Here's how the part is built. I have some questions about the finished solid (model axes, mm). Face numbers are marked on the shaded views. A direction names the side the tool comes from. Round coordinates to 2 decimals unless told otherwise and drop trailing zeros. Write each loop counter-clockwise with the first axis right and the second up, starting at its lowest first coordinate (ties: lowest second). Pieces come first, ordered by that corner, then holes. Notation, with made-up numbers: (41.5, -30.5) -> (99.5, -30.5) arc R28 ccw to (99.5, 7.5) -> close; hole circle Ø5 at (45.25, 87). An arc over 180 degrees is marked (long way). Answer as CSV lines item,"result".
from build123d import *

# Parameters (mm, degrees)
BOSS_EXTRUDE2_DEPTH = 8
SKETCH3_R           = 1.25
CUT_EXTRUDE1_DEPTH  = 8
CUT_EXTRUDE2_DEPTH  = 8


with BuildPart() as part:
    # Sketch1 → Boss-Extrude2 (new body)
    with BuildSketch(Plane.XY):
        with BuildLine():
            Line((-29.531751908, 7.051775609), (-24.531751908, 7.051775609))
            Line((-24.531751908, 7.051775609), (-24.531751908, -3.948224391))
            Line((-24.531751908, -3.948224391), (-134.531751908, -3.948224391))
            Line((-134.531751908, -3.948224391), (-134.531751908, 4.051775609))
            Line((-134.531751908, 4.051775609), (-36.531751908, 4.051775609))
            ThreePointArc((-36.531751908, 4.051775609), (-35.117538345, 4.637562047), (-34.531751908, 6.051775609))
            Line((-34.531751908, 6.051775609), (-34.531751908, 14.051775609))
            Line((-34.531751908, 14.051775609), (-29.531751908, 14.051775609))
            Line((-29.531751908, 14.051775609), (-29.531751908, 11.051775609))
            ThreePointArc((-29.531751908, 11.051775609), (-31.531751908, 9.051775609), (-29.531751908, 7.051775609))
        make_face()
    extrude(amount=BOSS_EXTRUDE2_DEPTH)

    # Sketch3 → Cut-Extrude1 (cut)
    with BuildSketch(Plane(origin=(0, 4.051775609, 0), x_dir=(1, 0, 0), z_dir=(0, 1, 0))):
        with Locations(Location((-130.531751908, -4, 0), (0, 0, 270))):
            Circle(SKETCH3_R)
    extrude(amount=-CUT_EXTRUDE1_DEPTH, mode=Mode.SUBTRACT)

    # Sketch4 → Cut-Extrude2 (cut)
    with BuildSketch(Plane(origin=(0, 4.051775609, 0), x_dir=(1, 0, 0), z_dir=(0, 1, 0))):
        with BuildLine():
            Line((-115.531751908, -2.5), (-95.531751908, -2.5))
            ThreePointArc((-95.531751908, -2.5), (-94.031751908, -4), (-95.531751908, -5.5))
            Line((-95.531751908, -5.5), (-115.531751908, -5.5))
            ThreePointArc((-115.531751908, -5.5), (-117.031751908, -4), (-115.531751908, -2.5))
        make_face()
    extrude(amount=-CUT_EXTRUDE2_DEPTH, mode=Mode.SUBTRACT)


solid = part.part
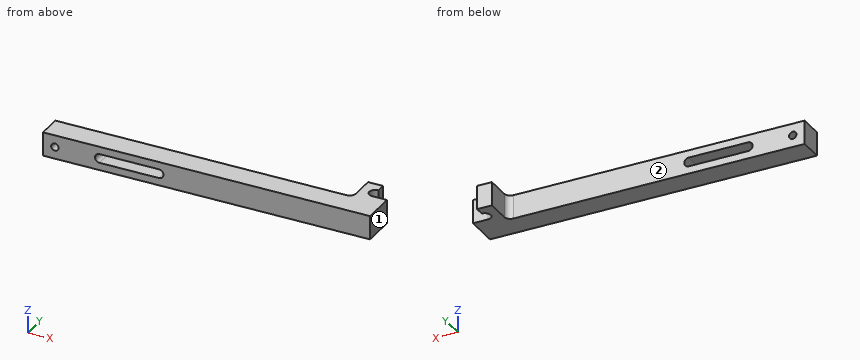
Item 1: Will these pins go through, and if not, where does the flat tip stop? pin 1 (2.5 mm diameter, centred on y = 13, z = 5.5, fed in from +X); pin 2 (4 mm diameter, centred on x = -26.5, z = 4, fed in from +Y); pin 3 (1 mm diameter, centred on y = 6, z = 3.5, fed in from -X).
Results found:
pin 1,"stops at x = -29.53"
pin 2,"stops at y = 7.05"
pin 3,"stops at x = -34.61"
Item 2: Suppose I cut it at C-C, the plane x = -71.5. List the corners of the cut face in (y, z) for me.
Results found:
outline,"(-3.95, 0) -> (4.05, 0) -> (4.05, 8) -> (-3.95, 8) -> close"
Item 3: Suppose I cut it at D-D, the plane y = 8.5. List the corners of the cut face in (x, z) for me.
Results found:
outline,"(-34.53, 0) -> (-31.45, 0) -> (-31.45, 8) -> (-34.53, 8) -> close"
Item 4: For the marked faces 1 and 2, which set-ups out of +Z, -Z, +X, -X, +Y, -Y let a thin tool reach every point of the face, with its end or its side?
Results found:
face 1,"+Z, -Z, +X, +Y, -Y"
face 2,"+Z, -Z, -X, +Y"
Item 5: Suppose I cut it at B-B, the plane y = 1. List the corners of the cut face in (x, z) for me, then the cut area to 3 significant figures.
Results found:
outline,"(-134.53, 0) -> (-24.53, 0) -> (-24.53, 8) -> (-134.53, 8) -> close; hole circle Ø2.5 at (-130.53, 4); hole (-115.53, 2.5) -> (-95.53, 2.5) arc R1.5 ccw to (-95.53, 5.5) -> (-115.53, 5.5) arc R1.5 ccw to start"
area,"808 mm²"
Item 6: Suppose I cut it at A-A, the plane z = 4. List the corners of the cut face in (x, y) for me.
Results found:
outline,"(-134.53, -3.95) -> (-131.78, -3.95) -> (-131.78, 4.05) -> (-134.53, 4.05) -> close; (-129.28, -3.95) -> (-117.03, -3.95) -> (-117.03, 4.05) -> (-129.28, 4.05) -> close; (-94.03, -3.95) -> (-24.53, -3.95) -> (-24.53, 7.05) -> (-29.53, 7.05) arc R2 cw to (-29.53, 11.05) -> (-29.53, 14.05) -> (-34.53, 14.05) -> (-34.53, 6.05) arc R2 cw to (-36.53, 4.05) -> (-94.03, 4.05) -> close"
Item 7: I need wall thicknesses on L1, parallel to X at y = 0, z = 4; L2, parallel to Z at x = -101.5, y = 4; L3, parallel to Y at x = -85.5, z = 3.5. Which ranges of each line are inside material? Lowest first, please.
Results found:
L1,"x = -134.53 to -131.78, -129.28 to -117.03, -94.03 to -24.53"
L2,"z = 0 to 2.5, 5.5 to 8"
L3,"y = -3.95 to 4.05"
